For this review, take the finished solid that the model builds, in its own axes (mm). Face numbers are marked on the shaded views. A direction names the side the tool comes from. Coordinates: 2 decimals unless noted, no trailing zeros. Loops run counter-clockwise (first coordinate to the right, second up) from the corner with the lowest first, then second, coordinate; pieces in that order, holes last.
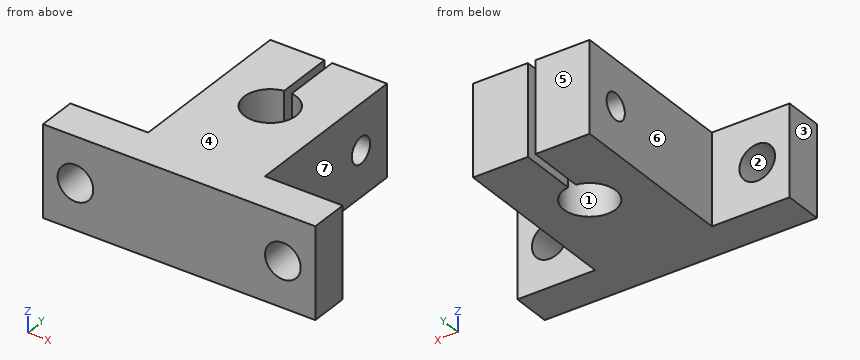
```python
from build123d import *

# Parameters (mm, degrees)
SKETCH_1_W          = 42
SKETCH_1_H          = 14
EXTRUDE_1_DEPTH     = 6
SKETCH_2_R          = 2.75
CUT_EXTRUDE_1_DEPTH = 30.423076981
SKETCH_3_W          = 18
SKETCH_3_H          = 14
EXTRUDE_2_DEPTH     = 26.8
SKETCH_4_R          = 4
CUT_EXTRUDE_2_DEPTH = 46.121439209
SKETCH_5_W          = 1.161233153
SKETCH_5_H          = 8.851007199
CUT_EXTRUDE_3_DEPTH = 46.121439209
SKETCH_7_R          = 2
CUT_EXTRUDE_4_DEPTH = 46.182443302


with BuildPart() as part:
    # 草图1 → 凸台-拉伸1 (new body)
    with BuildSketch(Plane(origin=(0, 0, 0), x_dir=(1, 0, 0), z_dir=(0, 1, 0))):
        with Locations((6.642436149, -1.100196464)):
            Rectangle(SKETCH_1_W, SKETCH_1_H)
    extrude(amount=EXTRUDE_1_DEPTH)

    # 草图2 → 切除-拉伸1 (cut, through all)
    with BuildSketch(Plane(origin=(0, 6, 0), x_dir=(1, 0, 0), z_dir=(0, 1, 0))):
        with Locations(Location((-9.357563851, -1.100196464, 0), (0, 0, 270))):
            Circle(SKETCH_2_R)
        with Locations(Location((22.642436149, -1.100196464, 0), (0, 0, 270))):
            Circle(SKETCH_2_R)
    extrude(amount=-CUT_EXTRUDE_1_DEPTH, mode=Mode.SUBTRACT)

    # 草图3 → 凸台-拉伸2 (add)
    with BuildSketch(Plane(origin=(0, 6, 0), x_dir=(1, 0, 0), z_dir=(0, 1, 0))):
        with Locations((6.642436149, -1.100196464)):
            Rectangle(SKETCH_3_W, SKETCH_3_H)
    extrude(amount=EXTRUDE_2_DEPTH)

    # 草图4 → 切除-拉伸2 (cut, through all)
    with BuildSketch(Plane.XY.offset(8.100196464)):
        with Locations((6.642436149, 20)):
            Circle(SKETCH_4_R)
    extrude(amount=-CUT_EXTRUDE_2_DEPTH, mode=Mode.SUBTRACT)

    # 草图5 → 切除-拉伸3 (cut, through all)
    with BuildSketch(Plane(origin=(0, 0, -5.899803536), x_dir=(-1, 0, 0), z_dir=(0, 0, -1))):
        with Locations((-6.586298571, 28.374496401)):
            Rectangle(SKETCH_5_W, SKETCH_5_H)
    extrude(amount=-CUT_EXTRUDE_3_DEPTH, mode=Mode.SUBTRACT)

    # 草图7 → 切除-拉伸4 (cut, through all)
    with BuildSketch(Plane.ZY.offset(2.357563851)):
        with Locations((1.100196464, 27.091605966)):
            Circle(SKETCH_7_R)
    extrude(amount=-CUT_EXTRUDE_4_DEPTH, mode=Mode.SUBTRACT)


solid = part.part
```
Q1. Wall thickness on probe 1 along X at (y, z) = (20, 4); probe 2 along X at (y, z) = (5, 3); probe 3 along X at (y, z) = (31, -1.25): over which ranges is each line inside the solid? List them lowest first.
Q2. Consider section A-A (y = 20). State the section outline as (x, z) points, then the cut area to 3 significant figures.
Q3. For pin 1 Ø1.5 at (y, z) = (24.5, -4) entering from +X; pin 2 Ø1.5 at (x, z) = (20, 0) entering from +Y; pin 3 Ø6.5 at (y, z) = (27.09, 1.1) entering from -X; pin 4 Ø5 at (x, z) = (14.5, 3.5) entering from -Y, all flat-tipped, find the tip position at first contact; note any pin that passes through.
Q4. Consider section B-B (z = -0.25). State the section outline as (x, y) points.
Q5. Consider section C-C (z = 6.5). State the section outline as (x, y) points, then the cut area to 3 significant figures.
Q6. The part is to be moulded in two halves that separate along X. For the marked faces 1, 2, 3 and 4, say which applies: +X half, -X half, draft (parallel to the pull), parting line (faces both ways), or undercut.
Q7. Consider section D-D (x = 1). State the section outline as (y, z) points, then the cut area to 3 significant figures.
Q8. Machinability: for the marked faces 5, 6 and 7, which of the approach directions +Z, -Z, +X, -X, +Y, -Y give a long, thin tool a straight path to every point of the face, cutting with its end or side? Answer none if there is none.
Model answer:
1. probe 1: x = -2.36 to 2.64, 10.64 to 15.64
1. probe 2: x = -14.36 to -11.35, -7.37 to 20.65, 24.63 to 27.64
1. probe 3: x = -2.36 to 6.01, 7.17 to 15.64
2. outline: (-2.36, -5.9) - (2.64, -5.9) - (2.64, 8.1) - (-2.36, 8.1) - close; (10.64, -5.9) - (15.64, -5.9) - (15.64, 8.1) - (10.64, 8.1) - close
2. area: 140 mm2
3. pin 1: stops at x = 15.64
3. pin 2: stops at y = 6
3. pin 3: stops at x = -2.36
3. pin 4: stops at y = 0
4. outline: (-14.36, 0) - (-11.75, 0) - (-11.75, 6) - (-14.36, 6) - close; (-6.96, 0) - (20.25, 0) - (20.25, 6) - (15.64, 6) - (15.64, 25.62) - (7.17, 25.62) - (7.17, 23.97) arc R4 cw (long way) to (6.01, 23.95) - (6.01, 25.62) - (-2.36, 25.62) - (-2.36, 6) - (-6.96, 6) - close; (-2.36, 28.57) - (6.01, 28.57) - (6.01, 32.8) - (-2.36, 32.8) - close; (7.17, 28.57) - (15.64, 28.57) - (15.64, 32.8) - (7.17, 32.8) - close; (25.04, 0) - (27.64, 0) - (27.64, 6) - (25.04, 6) - close
5. outline: (-14.36, 0) - (27.64, 0) - (27.64, 6) - (15.64, 6) - (15.64, 32.8) - (7.17, 32.8) - (7.17, 23.97) arc R4 cw (long way) to (6.01, 23.95) - (6.01, 32.8) - (-2.36, 32.8) - (-2.36, 6) - (-14.36, 6) - close
5. area: 674 mm2
6. face 1: undercut
6. face 2: undercut
6. face 3: -X half
6. face 4: draft
7. outline: (0, -5.9) - (32.8, -5.9) - (32.8, 8.1) - (0, 8.1) - close; hole circle Ø4 at (27.09, 1.1)
7. area: 447 mm2
8. face 5: +Z, -Z, +X, -X, +Y
8. face 6: +Z, -Z, -X, +Y
8. face 7: +Z, -Z, +X, +Y
